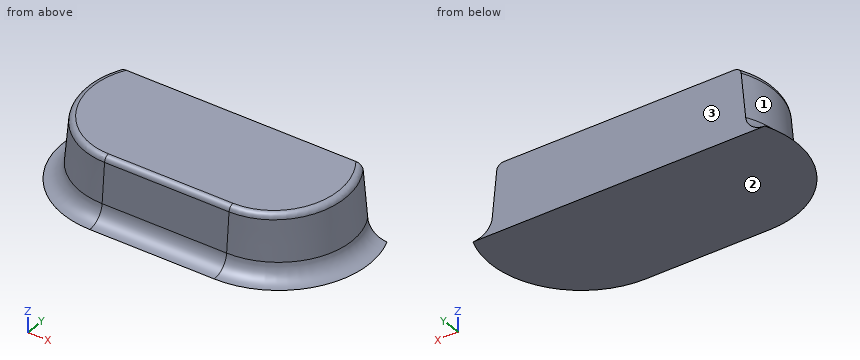
```python
from build123d import *

# Parameters (mm, degrees)
BOSS_EXTRUDE1_DEPTH = 12
BOSS_EXTRUDE1_TAPER = 5
SKETCH2_W           = 65.663584352
SKETCH2_H           = 13.360489219
CUT_EXTRUDE1_DEPTH  = 74.667326552
SKETCH3_W           = 72.132604944
SKETCH3_H           = 37.201111507
BOSS_EXTRUDE2_DEPTH = 10
FILLET1_R           = 3.5
SKETCH4_W           = 81.250289089
SKETCH4_H           = 16.618597718
CUT_EXTRUDE2_DEPTH  = 79.90066452
DRAFT2_ANGLE        = -4
FILLET3_R           = 1.2


with BuildPart() as part:
    # Sketch1 → Boss-Extrude1 (new body)
    with BuildSketch(Plane.XY):
        with BuildLine():
            Line((21.450148661, 8.816932272), (46.450148661, 8.816932272))
            ThreePointArc((46.450148661, 8.816932272), (61.450148661, 23.816932272), (46.450148661, 38.816932272))
            Line((46.450148661, 38.816932272), (21.450148661, 38.816932272))
            ThreePointArc((21.450148661, 38.816932272), (6.450148661, 23.816932272), (21.450148661, 8.816932272))
        make_face()
    extrude(amount=BOSS_EXTRUDE1_DEPTH, taper=BOSS_EXTRUDE1_TAPER)

    # Sketch2 → Cut-Extrude1 (cut, through all)
    with BuildSketch(Plane(origin=(0, 0, 0), x_dir=(-1, 0, 0), z_dir=(0, 0, -1))):
        with Locations((-32.000877842, 37.497176882)):
            Rectangle(SKETCH2_W, SKETCH2_H)
    extrude(amount=-CUT_EXTRUDE1_DEPTH, mode=Mode.SUBTRACT)

    # Sketch3 → Boss-Extrude2 (add)
    with BuildSketch(Plane(origin=(0, 0, 0), x_dir=(-1, 0, 0), z_dir=(0, 0, -1))):
        with Locations((-32.471221279, 19.407226217)):
            Rectangle(SKETCH3_W, SKETCH3_H)
    extrude(amount=BOSS_EXTRUDE2_DEPTH)

    # Fillet1
    fillet1_edges = [part.edges().sort_by_distance(p)[0] for p in [
        (59.295381239, 16.070965579, 0),
        (33.950148661, 8.816932272, 0),
        (8.604916082, 16.070965579, 0),
    ]]
    fillet(fillet1_edges, radius=FILLET1_R)

    # Sketch4 → Cut-Extrude2 (cut, through all)
    with BuildSketch(Plane.XZ.offset(-0.806670463)):
        with Locations((37.030063352, -8.309298859)):
            Rectangle(SKETCH4_W, SKETCH4_H)
    extrude(amount=-CUT_EXTRUDE2_DEPTH, mode=Mode.SUBTRACT)

    # Draft2
    draft2_faces = [part.faces().sort_by_distance(p)[0] for p in [
        (33.950148661, 20.873226907, 12),
    ]]
    draft(draft2_faces, Plane.ZX.offset(9.866796234), DRAFT2_ANGLE)

    # Fillet3
    fillet3_edges = [part.edges().sort_by_distance(p)[0] for p in [
        (58.506945165, 16.885570637, 12.490800518),
        (33.950148661, 9.866796234, 12),
        (9.393352156, 16.885570637, 12.490800518),
    ]]
    fillet(fillet3_edges, radius=FILLET3_R)


solid = part.part
```
Work out the finished part from the listing and answer in its coordinate system (mm). Face numbers are marked on the shaded views. Coordinates: 2 decimals unless noted, no trailing zeros. Write each loop counter-clockwise with the first axis right and the second up, starting at its lowest first coordinate (ties: lowest second). Pieces come first, ordered by that corner, then holes. Notation, with made-up numbers: (73, -16.75) - (101, -16.75) arc R19 cw to (101, -7.75) - close; hole circle Ø9 at (33, 21.25). An arc over 180 degrees is marked (long way). Answer as a JSON object with one key per item and string values.
Q1. Find section C-C (z = 9.25). Write down the section's boundary in (x, y), plus the area to 3 significant figures.
Results list:
{"outline": "(9.11, 30.82) arc R14.19 ccw to (21.45, 9.63) - (46.45, 9.63) arc R14.19 ccw to (58.79, 30.82) - close", "area": "1,040 mm^2"}
Q2. Find section A-A (x = 30). Write down the section's boundary in (y, z).
Results list:
{"outline": "(5.61, 0) - (30.82, 0) - (30.82, 13.46) - (10.89, 12.07) arc R1.2 ccw to (9.78, 10.98) - (9.1, 3.19) arc R3.5 cw to start"}
Q3. For a pull along Z with two mould halves and no side action, classify the marked faces 1, 2 and 3 as pulls with the +Z half, pulls with the -Z half, needs draft (parallel to the pull), parting line crosses it, or undercut.
Results list:
{"face 1": "pulls with the +Z half", "face 2": "pulls with the -Z half", "face 3": "needs draft"}
Q4. Find section B-B (z = 6.25). Write down the section's boundary in (x, y).
Results list:
{"outline": "(8.81, 30.82) arc R14.45 ccw to (21.45, 9.36) - (46.45, 9.36) arc R14.45 ccw to (59.1, 30.82) - close"}
Q5. Consider L1, parallel to X at y = 27, z = 10.5; L2, parallel to X at y = 18.5, z = 1.5; L3, parallel to Z at x = 8, y = 17.25. Determine where each line is inside the solid, lowest interval first. Write a range as from..to.
Results list:
{"L1": "x = 7.73..60.17", "L2": "x = 7.07..60.83", "L3": "z = 0..2.17"}
Q6. Given pin 1 Ø5 at (x, z) = (17, 5.5) entering from -Y; pin 2 Ø1 at (y, z) = (12.5, 2.5) entering from -X; pin 3 Ø8 at (y, z) = (25.5, 6.5) entering from +X, each flat-ended and moving along its own axis, determine where each tip first touches the part or whether it passes through.
Results list:
{"pin 1": "stops at y = 9.37", "pin 2": "stops at x = 11.22", "pin 3": "stops at x = 61.25"}
